The model under review builds one solid part; all positions refer to its coordinate system, in mm. Face numbers are marked on the shaded views. A direction names the side the tool comes from. Coordinates: 2 decimals unless noted, no trailing zeros. Write each loop counter-clockwise with the first axis right and the second up, starting at its lowest first coordinate (ties: lowest second). Pieces come first, ordered by that corner, then holes.
1) Add section A-A, the plane z = 0. State the section outline as (x, y) points, then the cut area to 3 significant figures.
2) Machinability: for the marked faces 5, 6 and 7, which of the approach directions +Z, -Z, +X, -X, +Y, -Y give a long, thin tool a straight path to every point of the face, cutting with its end or side? Answer none if there is none.
3) Add section B-B, the plane y = -4. State the section outline as (x, z) points (3 decimals), then the cut area to 3 significant figures.
4) For line 1 (Y direction, x = -4, z = -13.5); line 2 (X direction, y = 2, z = 0); line 3 (Y direction, x = 1, z = -5), list the stretches that pass through material, from the lowest coordinate up.
5) Add section C-C, the plane z = -13.25. State the section outline as (x, y) points, then the cut area to 3 significant figures.
6) For P1, Ø10, axis at x = 2.5, z = -9, coming from the +Y side; P2, Ø1, axis at y = -7, z = 4.5, coming from the -X side; P3, Ø1, axis at x = 2, y = -3.5, coming from the +Z side; P4, Ø5, axis at x = 1, z = -0.5, coming from the -Y side, all flat-tipped, find the tip position at first contact; note any pin that passes through.
7) Mouldability with a two-part tool opening along Y and no side actions: class the marked faces 1, 2, 3 and 4 as released by +Y, released by -Y, zero draft, split by the parting line, or undercut.
from build123d import *

# Parameters (mm, degrees)
CUT_EXTRUDE1_DEPTH = 11
CUT_EXTRUDE3_DEPTH = 5
FILLET1_R          = 0.5
FILLET3_R          = 0.5
CHAMFER2_SIZE      = 1
SKETCH12_R         = 1.4
CUT_EXTRUDE7_DEPTH = 5


with BuildPart() as part:
    # Sketch2 → Revolve1 (revolve)
    with BuildSketch(Plane(origin=(0, 0, 0), x_dir=(0, 0, -1), z_dir=(1, 0, 0))):
        Polygon((-2.5, 0), (-19.75, 0), (-19.75, -10), (-8.75, -10), (-8.75, -7), (-15.75, -7), (-15.75, -5), (-1.5, -5), (-1.5, 6), (-2.5, 6), (-3, 5), (-2.5, 5), (-2.5, 2), (-3, 1), (-2.5, 1), align=None)
    revolve(axis=Axis((0, 7.880012575, 0), (0, -1, 0)))

    # Sketch3 → Cut-Extrude1 (cut, through all)
    with BuildSketch(Plane(origin=(0, 0, 0), x_dir=(1, 0, 0), z_dir=(0, 1, 0))):
        with BuildLine():
            ThreePointArc((-10.703712775, -5.424991506), (-12, 0), (-10.703712775, 5.424991506))
            Line((-10.703712775, 5.424991506), (-5, 16.678631853))
            ThreePointArc((-5, 16.678631853), (-2.933994828, 18.920833005), (-3.1e-08, 19.75))
            ThreePointArc((-3.1e-08, 19.75), (-19.75, -1.6e-08), (0, -19.75))
            ThreePointArc((0, -19.75), (-2.933994815, -18.920833013), (-5, -16.678631853))
            Line((-5, -16.678631853), (-10.703712775, -5.424991506))
        make_face()
        with BuildLine():
            ThreePointArc((19.75, 0), (13.965358917, 13.965358939), (-3.1e-08, 19.75))
            ThreePointArc((-3.1e-08, 19.75), (2.933994802, 18.920833021), (5, 16.678631853))
            Line((5, 16.678631853), (10.703712775, 5.424991506))
            ThreePointArc((10.703712775, 5.424991506), (12, 0), (10.703712775, -5.424991506))
            Line((10.703712775, -5.424991506), (5, -16.678631853))
            ThreePointArc((5, -16.678631853), (2.933994815, -18.920833013), (0, -19.75))
            ThreePointArc((0, -19.75), (13.965358928, -13.965358928), (19.75, 0))
        make_face()
    extrude(amount=-CUT_EXTRUDE1_DEPTH, mode=Mode.SUBTRACT)

    # Sketch5 → Cut-Extrude3 (cut)
    with BuildSketch(Plane.XZ.offset(10)):
        with BuildLine():
            Line((-5.884741508, -8.695965581), (-11.34632201, -5))
            ThreePointArc((-11.34632201, -5), (-14, 0), (-11.34632201, 5))
            Line((-11.34632201, 5), (-5.884741508, 8.695965581))
            ThreePointArc((-5.884741508, 8.695965581), (0, 10.5), (5.884741508, 8.695965581))
            Line((5.884741508, 8.695965581), (11.34632201, 5))
            ThreePointArc((11.34632201, 5), (14, 0), (11.34632201, -5))
            Line((11.34632201, -5), (5.884741508, -8.695965581))
            ThreePointArc((5.884741508, -8.695965581), (0, -10.5), (-5.884741508, -8.695965581))
        make_face()
    extrude(amount=-CUT_EXTRUDE3_DEPTH, mode=Mode.SUBTRACT)

    # Fillet1
    fillet1_edges = [part.edges().sort_by_distance(p)[0] for p in [
        (-6.091971401, -6, -14.524131108),
        (-6.091971401, -6, 14.524131108),
        (6.091971401, -6, -14.524131108),
        (6.091971401, -6, 14.524131108),
        (10.696094588, -8.5, -5.440022476),
        (10.696094588, -8.5, 5.440022476),
        (-10.696094588, -8.5, 5.440022476),
        (-10.696094588, -8.5, -5.440022476),
    ]]
    fillet(fillet1_edges, radius=FILLET1_R)

    # Fillet3
    fillet3_edges = [part.edges().sort_by_distance(p)[0] for p in [
        (0, 0, -2.5),
    ]]
    fillet(fillet3_edges, radius=FILLET3_R)

    # Chamfer2
    chamfer2_edges = [part.edges().sort_by_distance(p)[0] for p in [
        (0, 0, 19.75),
        (-7.851856387, 0, 11.051811679),
        (-12, 0, 0),
        (-7.851856387, 0, -11.051811679),
        (0, 0, -19.75),
        (7.851856387, 0, 11.051811679),
        (7.851856387, 0, -11.051811679),
        (12, 0, 0),
    ]]
    chamfer(chamfer2_edges, length=CHAMFER2_SIZE)

    # Sketch12 → Cut-Extrude7 (cut)
    with BuildSketch(Plane.XZ.offset(10)):
        with Locations((0, -13.25)):
            Circle(SKETCH12_R)
        with Locations((0, 13.25)):
            Circle(SKETCH12_R)
    extrude(amount=-CUT_EXTRUDE7_DEPTH, mode=Mode.SUBTRACT)


solid = part.part
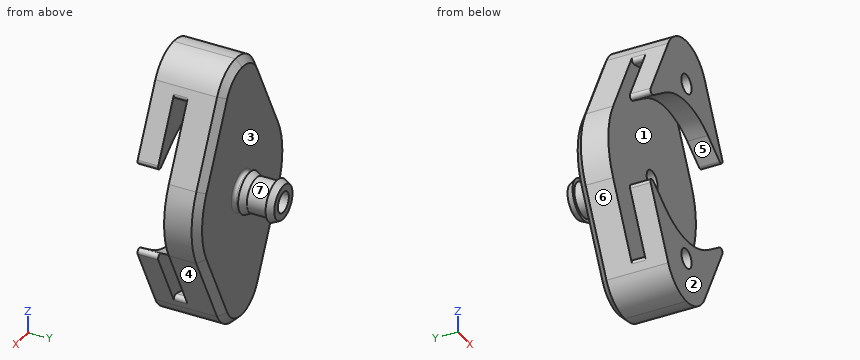
Geometry results:
1. outline: (-12, -5) - (-1.5, -5) - (-1.5, 6) - (-2.5, 6) - (-3, 5) - (-2.5, 5) - (-2.5, 2) - (-3, 1) - (-2.5, 1) - (-2.5, 0.5) arc R0.5 cw to (-3, 0) - (-11, 0) - (-12, -1) - close; (1.5, -5) - (12, -5) - (12, -1) - (11, 0) - (3, 0) arc R0.5 cw to (2.5, 0.5) - (2.5, 1) - (3, 1) - (2.5, 2) - (2.5, 5) - (3, 5) - (2.5, 6) - (1.5, 6) - close
1. area: 117 mm2
2. face 5: -Y
2. face 6: -Z, -X, +Y, -Y
2. face 7: none
3. outline: (-10.704, -5.425) - (-5, -16.679) arc R5.606 ccw to (5, -16.679) - (10.704, -5.425) arc R12 ccw to (10.704, 5.425) - (5, 16.679) arc R5.606 ccw to (-5, 16.679) - (-10.704, 5.425) arc R12 ccw to start; hole circle Ø3 at (0, 0)
3. area: 642 mm2
4. line 1: y = -10 to -7, -5 to 0
4. line 2: x = -2.5 to -1.5, 1.5 to 2.5
4. line 3: y = -5 to 0
5. outline: (-6.74, -10) - (-1.4, -10) - (-1.4, -7) - (-6.74, -7) - close; (-6.74, -5) - (6.74, -5) - (6.74, -1) - (5.62, 0) - (-5.62, 0) - (-6.74, -1) - close; (1.4, -10) - (6.74, -10) - (6.74, -7) - (1.4, -7) - close
5. area: 98.3 mm2
6. P1: stops at y = 0
6. P2: passes through
6. P3: stops at z = 19.55
6. P4: stops at y = -5
7. face 1: undercut
7. face 2: released by -Y
7. face 3: released by +Y
7. face 4: zero draft
